from build123d import *

# Parameters (mm, degrees)
F0_W     = 101.6
F0_H     = 76.2
F1_DEPTH = 152.4
F2_W     = 76.2
F2_H     = 25.4
F3_DEPTH = 70.104
F4_R     = 4.905682


with BuildPart() as f1:
    # F0 (on Top) → F1 (new body)
    with BuildSketch(Plane.XY):
        with Locations((38.523726, -72.381201)):
            Rectangle(F0_W, F0_H)
    extrude(amount=F1_DEPTH)

    # F2 (on face) → F3 (cut)
    with BuildSketch(Plane.XZ.offset(110.481201)):
        with Locations((38.523726, 129.54)):
            Rectangle(F2_W, F2_H)
        with Locations((38.523726, 93.98)):
            Rectangle(F2_W, F2_H)
        with Locations((38.523726, 58.42)):
            Rectangle(F2_W, F2_H)
        with Locations((38.523726, 22.86)):
            Rectangle(F2_W, F2_H)
    extrude(amount=-F3_DEPTH, mode=Mode.SUBTRACT)

    # F4
    f4_edges = [f1.edges().sort_by_distance(p)[0] for p in [
        (38.523726, -34.281201, 152.4),
        (-12.276274, -72.381201, 152.4),
        (38.523726, -110.481201, 152.4),
        (89.323726, -72.381201, 152.4),
        (89.323726, -110.481201, 76.2),
        (89.323726, -34.281201, 76.2),
        (89.323726, -72.381201, 0),
        (38.523726, -110.481201, 0),
        (38.523726, -34.281201, 0),
        (-12.276274, -34.281201, 76.2),
        (-12.276274, -110.481201, 76.2),
        (-12.276274, -72.381201, 0),
    ]]
    fillet(f4_edges, radius=F4_R)


solid = f1.part
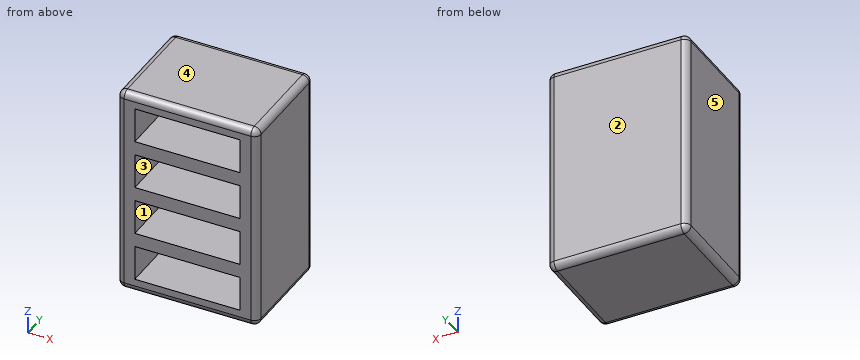
Design review of the part built by this model. Coordinates are the model's own, in mm. Face numbers are marked on the shaded views. A direction names the side the tool comes from. Round coordinates to 2 decimals unless told otherwise and drop trailing zeros. Order: outer loops, then holes, each group sorted by start corner. A loop starts at its lowest first (then second) coordinate and runs counter-clockwise, first axis right, second up.
1) Machinability: for the marked faces 1 and 2, which of the approach directions +Z, -Z, +X, -X, +Y, -Y give a long, thin tool a straight path to every point of the face, cutting with its end or side? Answer none if there is none.
The answers:
face 1: -Y
face 2: +Z, -Z, +X, -X, +Y
2) Draft analysis for pull direction Z (two halves, no side actions). For the marked faces 3, 4 and 5, state which applies: released by +Z, released by -Z, zero draft, split by the parting line, or undercut.
The answers:
face 3: undercut
face 4: released by +Z
face 5: zero draft
3) Consider section C-C (y = -88.5). State the section outline as (x, z) points, plus the area to 3 significant figures.
The answers:
outline: (-12.28, 4.91) arc R4.91 ccw to (-7.37, 0) - (84.42, 0) arc R4.91 ccw to (89.32, 4.91) - (89.32, 147.49) arc R4.91 ccw to (84.42, 152.4) - (-7.37, 152.4) arc R4.91 ccw to (-12.28, 147.49) - close; hole (0.42, 10.16) - (76.62, 10.16) - (76.62, 35.56) - (0.42, 35.56) - close; hole (0.42, 45.72) - (76.62, 45.72) - (76.62, 71.12) - (0.42, 71.12) - close; hole (0.42, 81.28) - (76.62, 81.28) - (76.62, 106.68) - (0.42, 106.68) - close; hole (0.42, 116.84) - (76.62, 116.84) - (76.62, 142.24) - (0.42, 142.24) - close
area: 7,720 mm2
4) Consider section A-A (x = 33). State the section outline as (y, z) points.
The answers:
outline: (-110.48, 4.91) arc R4.91 ccw to (-105.58, 0) - (-39.19, 0) arc R4.91 ccw to (-34.28, 4.91) - (-34.28, 147.49) arc R4.91 ccw to (-39.19, 152.4) - (-105.58, 152.4) arc R4.91 ccw to (-110.48, 147.49) - (-110.48, 142.24) - (-40.38, 142.24) - (-40.38, 116.84) - (-110.48, 116.84) - (-110.48, 106.68) - (-40.38, 106.68) - (-40.38, 81.28) - (-110.48, 81.28) - (-110.48, 71.12) - (-40.38, 71.12) - (-40.38, 45.72) - (-110.48, 45.72) - (-110.48, 35.56) - (-40.38, 35.56) - (-40.38, 10.16) - (-110.48, 10.16) - close
5) Consider section B-B (z = 52.5). State the section outline as (x, y) points, plus the area to 3 significant figures.
The answers:
outline: (-12.28, -105.58) arc R4.91 ccw to (-7.37, -110.48) - (0.42, -110.48) - (0.42, -40.38) - (76.62, -40.38) - (76.62, -110.48) - (84.42, -110.48) arc R4.91 ccw to (89.32, -105.58) - (89.32, -39.19) arc R4.91 ccw to (84.42, -34.28) - (-7.37, -34.28) arc R4.91 ccw to (-12.28, -39.19) - close
area: 2,380 mm2
6) For L1, parallel to Z at x = 37.5, y = -97; L2, parallel to X at y = -100, z = 137.5; L3, parallel to Y at x = 55, z = 52, list the stretches that pass through material, from the lowest coordinate up.
The answers:
L1: z = 0 to 10.16, 35.56 to 45.72, 71.12 to 81.28, 106.68 to 116.84, 142.24 to 152.4
L2: x = -12.28 to 0.42, 76.62 to 89.32
L3: y = -40.38 to -34.28
7) Clearance check with a flat-ended pin moving along its axis: pin 1 Ø7.5 at (x, z) = (53, 93.5) entering from -Y. State where the tip first meets the part, or that it passes through.
The answers:
pin 1: stops at y = -40.38
